from build123d import *

# Parameters (mm, degrees)
SKETCH_1_R          = 1.6
EXTRUDE_1_DEPTH     = 3
EXTRUDE_2_DEPTH     = 16
SKETCH_4_R          = 1.6
CUT_EXTRUDE_2_DEPTH = 38.973677807
FILLET_1_R          = 3


with BuildPart() as part:
    # 草图1 → 凸台-拉伸1 (new body)
    with BuildSketch(Plane(origin=(0, 0, 0), x_dir=(1, 0, 0), z_dir=(0, 1, 0))):
        Polygon((0, 5), (19.199124483, 20), (25.779802397, 20), (25.779802397, 0), (0, 0), align=None)
        with Locations(Location((20.206855342, 10, 0), (0, 0, 270))):
            Circle(SKETCH_1_R, mode=Mode.SUBTRACT)
    extrude(amount=EXTRUDE_1_DEPTH)

    # 草图2 → 凸台-拉伸2 (add)
    with BuildSketch(Plane(origin=(0, 3, 0), x_dir=(1, 0, 0), z_dir=(0, 1, 0))):
        Polygon((3.86182986, 8.017192162), (7.239873376, 3.69349363), (19.191382346, 13.031035803), (15.81333883, 17.354734335), align=None)
    extrude(amount=EXTRUDE_2_DEPTH)

    # 草图4 → 切除-拉伸2 (cut, through all)
    with BuildSketch(Plane(origin=(-2.425739316, 0, -3.104804739), x_dir=(-0.7880107536067209, 0, 0.6156614753256597), z_dir=(-0.6156614753256597, 0, -0.7880107536067209))):
        with Locations((-15.562381102, 10.681901231)):
            Circle(SKETCH_4_R)
    extrude(amount=-CUT_EXTRUDE_2_DEPTH, mode=Mode.SUBTRACT)

    # 圆角1
    fillet_1_edges = [part.edges().sort_by_distance(p)[0] for p in [
        (5.550851618, 19, -5.855342896),
        (17.502360588, 19, -15.192885069),
        (25.779802397, 1.5, -20),
        (0, 1.5, 0),
        (25.779802397, 1.5, 0),
    ]]
    fillet(fillet_1_edges, radius=FILLET_1_R)


solid = part.part
Geometry check sheet. Reference: the model listing, model coordinates, mm. A direction names the side the tool comes from. Coordinates: 2 decimals unless noted, no trailing zeros. Order: outer loops, then holes, each group sorted by start corner. A loop starts at its lowest first (then second) coordinate and runs counter-clockwise, first axis right, second up. Notation, with made-up numbers: (82, 71.5) - (92, 71.5) arc R24 cw to (92, 110.5) - close; hole circle Ø4 at (82, 24). An arc over 180 degrees is marked (long way). Answer in a Markdown table with one row per item. Add a question column.
1) Cross-section at B-B, the plane x = 2.25. Record the cut outline in (y, z), then the cut area to 3 significant figures.
2) Set-up check for faces 4 (the flat face through (5.527, 9.409, -5.886)), 5 (the flat face through (11.804, 10.888, -7.259)), 6 (the flat face through (17.53, 9.41, -15.16)): record each of +Z, -Z, +X, -X, +Y, -Y from which the full face is reachable in a straight line by a thin tool's end or side.
3) Material ranges on line 1 along Y through (x, z) = (19.75, -16); line 2 along X through (y, z) = (10, -11.5); line 3 along X through (y, z) = (1.85, -10), recorded low to high. Write a range as [from, to].
4) Gauge pin test, flat ends, axial feed: P1, Ø5, axis at x = 20.21, z = -10, coming from the -Y side; P2, Ø1, axis at y = 3, z = -18, coming from the +X side; P3, Ø2, axis at y = 16, z = -16.5, coming from the +X side; P4, Ø5, axis at x = 8, y = 8.5, coming from the -Z side. Record the tip position at first contact, or that the pin passes through.
5) Release check for a two-part mould opening along X. For faces 1 (the flat face through (0, 1, -4)), 2 (the flat face through (25.78, 1, -10)), 3 (the cylindrical face through (11.78, 9.12, -10.77)) record: +X half, -X half, draft (parallel to the pull), parting line (faces both ways), or undercut.
6) Cross-section at A-A, the plane y = 5. Record the cut outline in (x, z), then the cut area to 3 significant figures.
Check result:
| question | item | result |
|---|---|---|
| 1 | outline | (0, -6.76) - (3, -6.76) - (3, -0.1) - (0, -0.1) - close |
| 1 | area | 20.0 mm² |
| 2 | face 4 | +Z, -X, +Y |
| 2 | face 5 | +Z, +X, +Y |
| 2 | face 6 | -Z, +X, +Y |
| 3 | line 1 | y = [0, 3] |
| 3 | line 2 | x = [8.32, 8.93], [12.6, 17.23] |
| 3 | line 3 | x = [6.4, 18.61], [21.81, 25.78] |
| 4 | P1 | stops at y = 0 |
| 4 | P2 | stops at x = 25.74 |
| 4 | P3 | stops at x = 17.26 |
| 4 | P4 | stops at z = -13.2 |
| 5 | face 1 | -X half |
| 5 | face 2 | +X half |
| 5 | face 3 | undercut |
| 6 | outline | (3.86, -8.02) - (15.81, -17.35) - (19.19, -13.03) - (7.24, -3.69) - close |
| 6 | area | 83.2 mm² |
